Source: three-view drawing plus pictorial views. Frame: mm from the lowest corner of the part. Round coordinates to 2 decimals unless told otherwise and drop trailing zeros. Answer as CSV lines item,"result". Start each with the question number.
Q1. Section query A-A on z = 12.7. Give the number of separate pieces and of enclosed holes in the cut face, and give its area (3 significant figures).
Q2. Ray query, probe 1 along Z at (x, y) = (57.15, 1.1); probe 2 along Z at (x, y) = (48.5, 3); probe 3 along X at (y, z) = (1.75, 34). Return the intervals inside material, ascending.
Q3. First-contact query: pin 1 (1 mm diameter, centred on x = 61, y = 1, fed in from -Z); pin 2 (1.6 mm diameter, centred on x = 22, y = 1, fed in from +Z); pin 3 (1 mm diameter, centred on y = 2, z = 44.5, fed in from -X) (1 decimal). Flat tips, straight axial feed; report the tip coordinate or a pass-through.
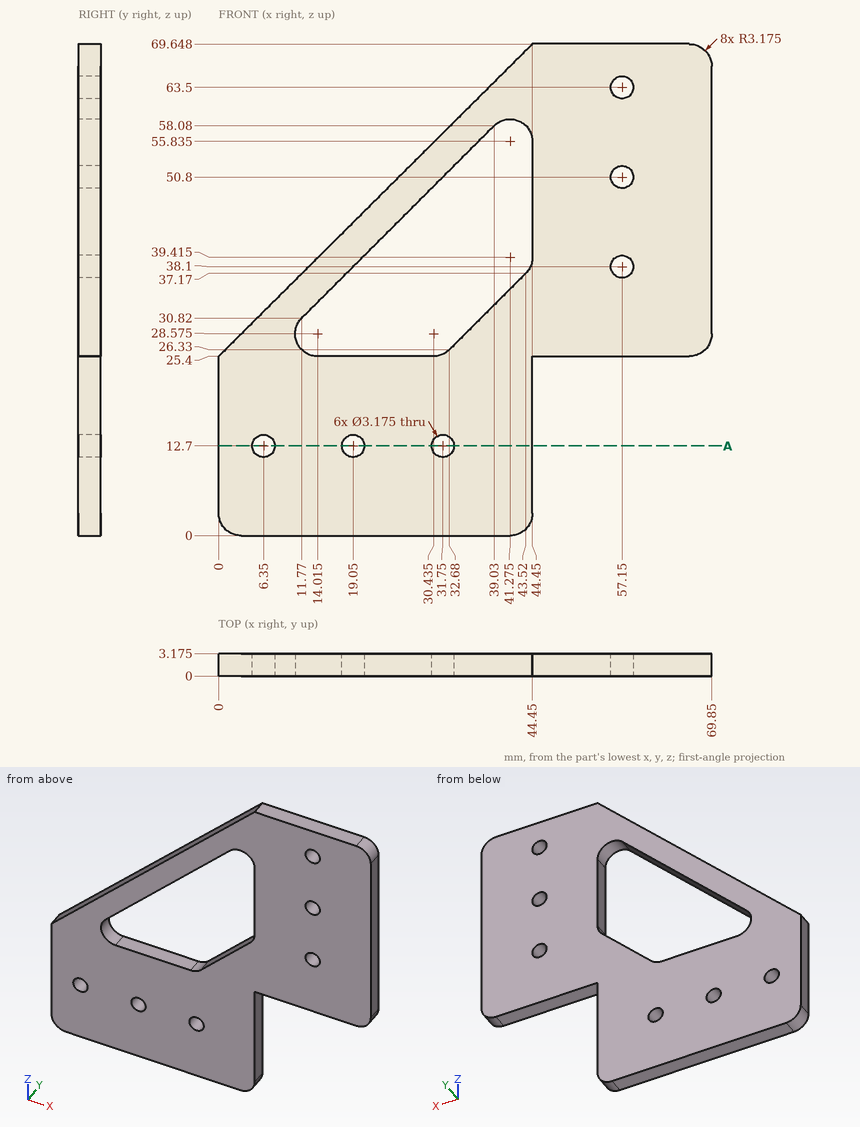
Entries:
1,separate pieces,"4"
1,enclosed holes,"0"
1,area,"111 mm^2"
2,probe 1,"z = 25.4 to 36.51, 39.69 to 49.21, 52.39 to 61.91, 65.09 to 69.65"
2,probe 2,"z = 25.4 to 69.65"
2,probe 3,"x = 8.64 to 14.95, 40.35 to 69.85"
3,pin 1,"stops at z = 25.4"
3,pin 2,"stops at z = 48.1"
3,pin 3,"stops at x = 18.7"
